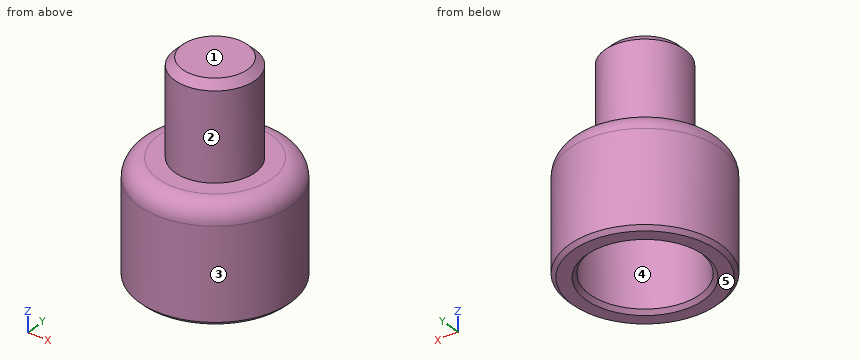
```python
from build123d import *

# Parameters (mm, degrees)
F0_R     = 20
F1_DEPTH = 30
F2_R     = 10.6
F3_DEPTH = 25
F5_R     = 14.55
F6_DEPTH = 22
F7_SIZE  = 2
F8_R     = 5
F9_SIZE  = 1


with BuildPart() as f1:
    # F0 (on Top) → F1 (new body)
    with BuildSketch(Plane.XY):
        Circle(F0_R)
    extrude(amount=-F1_DEPTH)

    # F2 (on Top) → F3 (join)
    with BuildSketch(Plane.XY):
        Circle(F2_R)
    extrude(amount=F3_DEPTH)

    # F5 (on offset) → F6 (cut)
    with BuildSketch(Plane(origin=(0, 0, -30), x_dir=(1, 0, 0), z_dir=(0, 0, -1))):
        Circle(F5_R)
    extrude(amount=-F6_DEPTH, mode=Mode.SUBTRACT)

    # F7
    f7_edges = [f1.edges().sort_by_distance(p)[0] for p in [
        (-10.6, 0, 25),
    ]]
    chamfer(f7_edges, length=F7_SIZE)

    # F8
    f8_edges = [f1.edges().sort_by_distance(p)[0] for p in [
        (-20, 0, 0),
    ]]
    fillet(f8_edges, radius=F8_R)

    # F9
    f9_edges = [f1.edges().sort_by_distance(p)[0] for p in [
        (-20, 0, -30),
        (-14.55, 0, -30),
    ]]
    chamfer(f9_edges, length=F9_SIZE)


solid = f1.part
```
The listing builds one solid part. Answer for the finished solid, in the listing's coordinates (mm). Face numbers are marked on the shaded views. A direction names the side the tool comes from. Coordinates: 2 decimals unless noted, no trailing zeros. Order: outer loops, then holes, each group sorted by start corner. A loop starts at its lowest first (then second) coordinate and runs counter-clockwise, first axis right, second up. Notation, with made-up numbers: M 31,-11.5 L 74,-11.5 A33 ccw 74,19.5 Z; hole C 66,49 d3. An arc over 180 degrees is marked long. Answer as a JSON object with one key per item and string values. Group by question number.
1. Determine the mould class of the marked faces 3, 4 and 5 for opening direction X: released by +X, released by -X, zero draft, split by the parting line, or undercut.
2. Section D-D on z = -17 is taken. Write down the section's boundary in (x, y), then the cut area to 3 significant figures.
3. Flat-ended cylindrical pins translate along their axes: P1, Ø5, axis at y = 11, z = 17, coming from the +X side; P2, Ø12, axis at x = 13, y = 11, coming from the +Z side; P3, Ø3, axis at x = 9, z = 11.5, coming from the -Y side. Find the tip coordinate at first contact, or state that the pin passes through.
4. Section A-A on y = 0 is taken. Write down the section's boundary in (x, z), then the cut area to 3 significant figures.
5. Section C-C on z = 15.5 is taken. Write down the section's boundary in (x, y).
6. Straight lines are drawn through the part: line 1 (Y direction, x = 0, z = -18.5); line 2 (Y direction, x = 8.5, z = -14); line 3 (Z direction, x = -0.5, y = -14.5). For each, find the intervals that lie inside material, in ascending order.
7. A tool of negligible diameter and unlimited length cuts with its end or side. For the marked faces 1 and 2, from which of +Z, -Z, +X, -X, +Y, -Y can it reach the whole face along a straight path? Write none if from no direction.
Values follow:
{
 "1": {"face 3": "split by the parting line", "face 4": "undercut", "face 5": "zero draft"},
 "2": {"outline": "C 0,0 d40; hole C 0,0 d29.1", "area": "592 mm2"},
 "3": {"P1": "x = 6.33", "P2": "z = 0", "P3": "y = -7.49"},
 "4": {"outline": "M -20,-29 L -19,-30 L -15.55,-30 L -14.55,-29 L -14.55,-8 L 14.55,-8 L 14.55,-29 L 15.55,-30 L 19,-30 L 20,-29 L 20,-5 A5 ccw 15,0 L 10.6,0 L 10.6,23 L 8.6,25 L -8.6,25 L -10.6,23 L -10.6,0 L -15,0 A5 ccw -20,-5 Z", "area": "1,070 mm2"},
 "5": {"outline": "C 0,0 d21.2"},
 "6": {"line 1": "-20 to -14.55, 14.55 to 20", "line 2": "-18.1 to -11.81, 11.81 to 18.1", "line 3": "-8 to 0"},
 "7": {"face 1": "+Z, +X, -X, +Y, -Y", "face 2": "+Z"}
}
